Build history of the part. All positions in model axes, mm. A direction names the side the tool comes from. Round coordinates to 2 decimals unless told otherwise and drop trailing zeros. Order: outer loops, then holes, each group sorted by start corner. A loop starts at its lowest first (then second) coordinate and runs counter-clockwise, first axis right, second up. Notation, with made-up numbers: (45, 10) -> (69, 10) arc R36 ccw to (69, 47) -> close; hole circle Ø8 at (77, -34). An arc over 180 degrees is marked (long way). Write item = value, one per line.
from build123d import *

# Parameters (mm, degrees)
F1_DEPTH = 75
F2_R     = 2


with BuildPart() as f1:
    # F0 (on Top) → F1 (new body)
    with BuildSketch(Plane.XY):
        with BuildLine():
            Line((35.5, 21.5), (-35.5, 21.5))
            ThreePointArc((-35.5, 21.5), (-39.035534, 20.035534), (-40.5, 16.5))
            Line((-40.5, 16.5), (-40.5, -16.5))
            ThreePointArc((-40.5, -16.5), (-39.035534, -20.035534), (-35.5, -21.5))
            Line((-35.5, -21.5), (35.5, -21.5))
            ThreePointArc((35.5, -21.5), (39.035534, -20.035534), (40.5, -16.5))
            Line((40.5, -16.5), (40.5, 16.5))
            ThreePointArc((40.5, 16.5), (39.035534, 20.035534), (35.5, 21.5))
        make_face()
    extrude(amount=F1_DEPTH)

    # F2
    f2_edges = [f1.edges().sort_by_distance(p)[0] for p in [
        (0, 21.5, 75),
        (-39.035534, 20.035534, 75),
        (-40.5, 0, 75),
        (-39.035534, -20.035534, 75),
        (0, -21.5, 75),
        (39.035534, -20.035534, 75),
        (40.5, 0, 75),
        (39.035534, 20.035534, 75),
        (0, 21.5, 0),
        (-39.035534, 20.035534, 0),
        (-40.5, 0, 0),
        (-39.035534, -20.035534, 0),
        (0, -21.5, 0),
        (39.035534, -20.035534, 0),
        (40.5, 0, 0),
        (39.035534, 20.035534, 0),
    ]]
    fillet(f2_edges, radius=F2_R)

    # F3 (on Front) → F4 (revolve)
    with BuildSketch(Plane.XZ):
        Polygon((38.769069, 74.981818), (40.5, 68.981818), (53.5, 68.981818), (53.5, 72.981818), align=None)
    revolve(axis=Axis((47, 0, 68.981818), (1, 0, 0)))


solid = f1.part
Q1. Which spindle directions (+Z, -Z, +X, -X, +Y, -Y) get a long thin tool onto all of the face, cutting with end or side? Do faces 1 (the face through (38.7, 0.23, 74.99)), 2 (the face through (0, 21.5, 37)). Say none if no direction does.
Check values:
face_1 = +Z, +X
face_2 = +Z, -Z, +X, -X, +Y
Q2. Flat gauge pin, fed straight in: pin 1 (2 mm diameter, centred on y = 16.5, z = 32, fed in from +X). Where does the tip first touch, or does it go through?
Check values:
pin_1 = 40.5
Q3. Cut at A-A, the plane y = 0. List the corners of the cut face in (x, z).
Check values:
outline = (-40.5, 2) arc R2 ccw to (-38.5, 0) -> (38.5, 0) arc R2 ccw to (40.5, 2) -> (40.5, 63.22) -> (53.5, 64.98) -> (53.5, 72.98) -> (38.77, 74.98) arc R2 ccw to (38.5, 75) -> (-38.5, 75) arc R2 ccw to (-40.5, 73) -> close
Q4. Cut at B-B, the plane z = 33. List the corners of the cut face in (x, y).
Check values:
outline = (-40.5, -16.5) arc R5 ccw to (-35.5, -21.5) -> (35.5, -21.5) arc R5 ccw to (40.5, -16.5) -> (40.5, 16.5) arc R5 ccw to (35.5, 21.5) -> (-35.5, 21.5) arc R5 ccw to (-40.5, 16.5) -> close
Q5. Probe probe 1 along X at (y, z) = (-13.5, 47); probe 2 along Z at (x, y) = (41, 4); probe 3 along X at (y, z) = (-18, 39.5). List the from-to ranges inside material, lowest first.
Check values:
probe_1 = -40.5 to 40.5
probe_2 = 64.93 to 73.04
probe_3 = -40.27 to 40.27
Q6. Cut at C-C, the plane y = 8. List the corners of the cut face in (x, z), and give its area (3 significant figures).
Check values:
outline = (-40.5, 2) arc R2 ccw to (-38.5, 0) -> (38.5, 0) arc R2 ccw to (40.5, 2) -> (40.5, 73) arc R2 ccw to (38.5, 75) -> (-38.5, 75) arc R2 ccw to (-40.5, 73) -> close
area = 6,070 mm²
